from build123d import *

# Parameters (mm, degrees)
ESQUISSE1_W                = 48
ESQUISSE1_H                = 24
EXTRUSION1_DEPTH           = 7.5
CONG_2_R                   = 5
CONG_5_R                   = 1
CONG_6_R                   = 1
ESQUISSE4_W                = 0.5
ESQUISSE4_H                = 18.982849842
EXTRUSION2_DEPTH           = 0.5
ESQUISSE5_R                = 0.25
EXTRUSION3_DEPTH           = 0.5
CHANFREIN1_SIZE            = 1
ESQUISSE10_R               = 2
EXTRUSION7_DEPTH           = 0.5
EXTRUSION7_DRAFT           = -45
EXTRUSION7_PROFILE_2_DEPTH = 0.5
EXTRUSION7_PROFILE_2_DRAFT = -45
ESQUISSE11_R               = 2.5
EXTRUSION8_DEPTH           = 0.5
EXTRUSION8_DRAFT           = -45


with BuildPart() as part:
    # Esquisse1 → Extrusion1 (new body)
    with BuildSketch(Plane(origin=(0, 0, 0), x_dir=(1, 0, 0), z_dir=(0, 1, 0))):
        with Locations((24, 12)):
            Rectangle(ESQUISSE1_W, ESQUISSE1_H)
    extrude(amount=EXTRUSION1_DEPTH)

    # Congé2
    cong_2_edges = [part.edges().sort_by_distance(p)[0] for p in [
        (0, 3.75, -24),
        (48, 3.75, -24),
        (48, 3.75, 0),
        (0, 3.75, 0),
    ]]
    fillet(cong_2_edges, radius=CONG_2_R)

    # Congé5
    cong_5_edges = [part.edges().sort_by_distance(p)[0] for p in [
        (48, 7.5, -12),
        (24, 7.5, 0),
        (0, 7.5, -12),
        (24, 7.5, -24),
        (1.464466094, 7.5, -22.535533906),
        (1.464466094, 7.5, -1.464466094),
        (46.535533906, 7.5, -22.535533906),
        (46.535533906, 7.5, -1.464466094),
    ]]
    fillet(cong_5_edges, radius=CONG_5_R)

    # Congé6
    cong_6_edges = [part.edges().sort_by_distance(p)[0] for p in [
        (48, 0, -12),
        (0, 0, -12),
        (24, 0, -24),
        (24, 0, 0),
        (1.464466094, 0, -22.535533906),
        (1.464466094, 0, -1.464466094),
        (46.535533906, 0, -22.535533906),
        (46.535533906, 0, -1.464466094),
    ]]
    fillet(cong_6_edges, radius=CONG_6_R)

    # Esquisse4 → Extrusion2 (cut)
    with BuildSketch(Plane(origin=(0, 7.5, 0), x_dir=(1, 0, 0), z_dir=(0, 1, 0))):
        with Locations((24, 12)):
            Rectangle(ESQUISSE4_W, ESQUISSE4_H)
    extrude(amount=-EXTRUSION2_DEPTH, mode=Mode.SUBTRACT)

    # Esquisse5 → Extrusion3 (cut)
    with BuildSketch(Plane(origin=(0, 7.5, 0), x_dir=(1, 0, 0), z_dir=(0, 1, 0))):
        with Locations((24, 21.491424921)):
            Circle(ESQUISSE5_R)
        with Locations((24, 2.508575079)):
            Circle(ESQUISSE5_R)
    extrude(amount=-EXTRUSION3_DEPTH, mode=Mode.SUBTRACT)

    # Chanfrein1
    # the kernel refuses this chamfer: 1 mm, written as the material it takes off along each edge
    with BuildSketch(Plane(origin=(24, 7.5, -21.491424921), x_dir=(1, 0, 0), z_dir=(0, 0, 1))) as chanfrein1_piece_1_section:
        Polygon((0.25 + CHANFREIN1_SIZE, 0), (0.25, -CHANFREIN1_SIZE), (0.25, 0), align=None)
    chanfrein1_piece_1 = revolve(axis=Axis((24, 7.5, -21.491424921), (0, 1, 0)), revolution_arc=180, mode=Mode.PRIVATE)
    chanfrein1_piece_1 = split(chanfrein1_piece_1, bisect_by=Plane(origin=(24, 7, -21.964580549), z_dir=(0, 1, 0)), keep=Keep.TOP, mode=Mode.PRIVATE)
    add(chanfrein1_piece_1, mode=Mode.SUBTRACT)
    with BuildSketch(Plane(origin=(24.25, 7.5, -21.491424921), x_dir=(0.9996219169112968, 0.02749587661058651, 0), z_dir=(0, 0, 1))) as chanfrein1_piece_2_section:
        Polygon((CHANFREIN1_SIZE * 0.999621916911, -CHANFREIN1_SIZE * 0.0274958766106), (-CHANFREIN1_SIZE * 0.0274958766106, -CHANFREIN1_SIZE * 0.999621916911), (0, 0), align=None)
    chanfrein1_piece_2 = extrude(amount=18.982849842, mode=Mode.PRIVATE)
    chanfrein1_piece_2 = split(chanfrein1_piece_2, bisect_by=Plane(origin=(24.643401084, 7, -12), z_dir=(0, 1, 0)), keep=Keep.TOP, mode=Mode.PRIVATE)
    add(chanfrein1_piece_2, mode=Mode.SUBTRACT)
    with BuildSketch(Plane(origin=(24, 7.5, -2.508575079), x_dir=(-1, 0, 0), z_dir=(0, 0, -1))) as chanfrein1_piece_3_section:
        Polygon((0.25 + CHANFREIN1_SIZE, 0), (0.25, -CHANFREIN1_SIZE), (0.25, 0), align=None)
    chanfrein1_piece_3 = revolve(axis=Axis((24, 7.5, -2.508575079), (0, 1, 0)), revolution_arc=180, mode=Mode.PRIVATE)
    chanfrein1_piece_3 = split(chanfrein1_piece_3, bisect_by=Plane(origin=(24, 7, -2.035419451), z_dir=(0, 1, 0)), keep=Keep.TOP, mode=Mode.PRIVATE)
    add(chanfrein1_piece_3, mode=Mode.SUBTRACT)
    with BuildSketch(Plane(origin=(23.75, 7.5, -2.508575079), x_dir=(-0.9996219169112968, 0.02749587661058651, 0), z_dir=(0, 0, -1))) as chanfrein1_piece_4_section:
        Polygon((CHANFREIN1_SIZE * 0.999621916911, -CHANFREIN1_SIZE * 0.0274958766106), (-CHANFREIN1_SIZE * 0.0274958766106, -CHANFREIN1_SIZE * 0.999621916911), (0, 0), align=None)
    chanfrein1_piece_4 = extrude(amount=18.982849842, mode=Mode.PRIVATE)
    chanfrein1_piece_4 = split(chanfrein1_piece_4, bisect_by=Plane(origin=(23.356598916, 7, -12), z_dir=(0, 1, 0)), keep=Keep.TOP, mode=Mode.PRIVATE)
    add(chanfrein1_piece_4, mode=Mode.SUBTRACT)


with BuildPart() as extrusion7_tool:
    # Esquisse10 → Extrusion7 (with draft: the straight prism first)
    with BuildSketch(Plane(origin=(0, 7.5, 0), x_dir=(1, 0, 0), z_dir=(0, 1, 0))):
        with Locations((7, 17)):
            Circle(ESQUISSE10_R)
    extrude(amount=-EXTRUSION7_DEPTH)
    # Extrusion7: the draft: its side faces are tilted about the plane it starts from
    extrusion7_sides = [extrusion7_tool.faces().sort_by_distance(p)[0] for p in [
        (5, 7.25, -17),
    ]]
    draft(extrusion7_sides, Plane(origin=(0, 7.5, 0), x_dir=(1, 0, 0), z_dir=(0, 1, 0)), EXTRUSION7_DRAFT)


with BuildPart() as part_1:
    add(part.part)

    # Extrusion7: cut by extrusion7_tool
    add(extrusion7_tool.part, mode=Mode.SUBTRACT)


with BuildPart() as extrusion7_profile_2_tool:
    # Esquisse10 → Extrusion7 profile 2 (with draft: the straight prism first)
    with BuildSketch(Plane(origin=(0, 7.5, 0), x_dir=(1, 0, 0), z_dir=(0, 1, 0))):
        with Locations((16.75, 7)):
            Circle(ESQUISSE10_R)
    extrude(amount=-EXTRUSION7_PROFILE_2_DEPTH)
    # Extrusion7 profile 2: the draft: its side faces are tilted about the plane it starts from
    extrusion7_profile_2_sides = [extrusion7_profile_2_tool.faces().sort_by_distance(p)[0] for p in [
        (14.75, 7.25, -7),
    ]]
    draft(extrusion7_profile_2_sides, Plane(origin=(0, 7.5, 0), x_dir=(1, 0, 0), z_dir=(0, 1, 0)), EXTRUSION7_PROFILE_2_DRAFT)


with BuildPart() as part_2:
    add(part_1.part)

    # Extrusion7 profile 2: cut by extrusion7_profile_2_tool
    add(extrusion7_profile_2_tool.part, mode=Mode.SUBTRACT)


with BuildPart() as extrusion8_tool:
    # Esquisse11 → Extrusion8 (with draft: the straight prism first)
    with BuildSketch(Plane(origin=(0, 7.5, 0), x_dir=(1, 0, 0), z_dir=(0, 1, 0))):
        with Locations((36, 12)):
            Circle(ESQUISSE11_R)
    extrude(amount=-EXTRUSION8_DEPTH)
    # Extrusion8: the draft: its side faces are tilted about the plane it starts from
    extrusion8_sides = [extrusion8_tool.faces().sort_by_distance(p)[0] for p in [
        (33.5, 7.25, -12),
    ]]
    draft(extrusion8_sides, Plane(origin=(0, 7.5, 0), x_dir=(1, 0, 0), z_dir=(0, 1, 0)), EXTRUSION8_DRAFT)


with BuildPart() as part_3:
    add(part_2.part)

    # Extrusion8: cut by extrusion8_tool
    add(extrusion8_tool.part, mode=Mode.SUBTRACT)


solid = part_3.part
Read the model definition and answer for the solid it produces. Units are mm, in the model's axes. A direction names the side the tool comes from. Round coordinates to 2 decimals unless told otherwise and drop trailing zeros. Write each loop counter-clockwise with the first axis right and the second up, starting at its lowest first coordinate (ties: lowest second). Pieces come first, ordered by that corner, then holes.
Q1. A flat-ended cylindrical pin translates along its axis: P1, Ø1.6, axis at x = 24, z = -15.5, coming from the +Y side. Find the tip coordinate at first contact, or state that the pin passes through.
Values:
P1: stops at y = 7.05
Q2. Straight lines are drawn through the part: line 1 (Y direction, x = 16.5, z = -7.75); line 2 (Y direction, x = 24.5, z = -1.75); line 3 (Z direction, x = 46.5, y = 3). For each, find the intervals that lie inside material, in ascending order.
Values:
line 1: y = 0 to 7
line 2: y = 0 to 7.16
line 3: z = -22.57 to -1.43
Q3. A tool of negligible diameter and unlimited length cuts with its end or side. For faces 5 (the face through (17, 7, -7)), 6 (the face through (23.734, 7.215, -23.699)), from which of +Z, -Z, +X, -X, +Y, -Y can it reach the whole face along a straight path? Write none if from no direction.
Values:
face 5: +Y
face 6: -Z, +X, -X, +Y
Q4. Find section B-B on x = 36. Determine the outline of the cut face in (y, z).
Values:
outline: (0, -23) arc R1 ccw to (1, -24) - (6.5, -24) arc R1 ccw to (7.5, -23) - (7.5, -14.5) - (7, -14) - (7, -10) - (7.5, -9.5) - (7.5, -1) arc R1 ccw to (6.5, 0) - (1, 0) arc R1 ccw to (0, -1) - close
Q5. Find section A-A on y = 2. Determine the outline of the cut face in (x, z).
Values:
outline: (0, -19) arc R5 ccw to (5, -24) - (43, -24) arc R5 ccw to (48, -19) - (48, -5) arc R5 ccw to (43, 0) - (5, 0) arc R5 ccw to (0, -5) - close
Q6. The mould has two halves that part along X. Classify faces 1 (the face through (47, 4, -22)), 2 (the face through (23.734, 0.285, -23.699)), 3 (the face through (23.98, 7.14, -1.62)), 4 (the face through (1, 4, -2)): released by +X, released by -X, zero draft, split by the parting line, or undercut.
Values:
face 1: released by +X
face 2: zero draft
face 3: undercut
face 4: released by -X
